```python
from build123d import *

# Parameters (mm, degrees)
SKETCH1_W           = 25.0000008
SKETCH1_H           = 24.00000026
SKETCH1_W_2         = 17.000000544
SKETCH1_H_2         = 16.000000004
BOSS_EXTRUDE1_DEPTH = 2.54
SKETCH2_R           = 1.000000032
CUT_EXTRUDE1_DEPTH  = 2.54


with BuildPart() as part:
    # Sketch1 → Boss-Extrude1 (new body)
    with BuildSketch(Plane.XY):
        Rectangle(SKETCH1_W, SKETCH1_H)
        Rectangle(SKETCH1_W_2, SKETCH1_H_2, mode=Mode.SUBTRACT)
    extrude(amount=BOSS_EXTRUDE1_DEPTH)

    # Sketch2 → Cut-Extrude1 (cut)
    with BuildSketch(Plane.XY.offset(0.635)):
        with Locations((-10.500000336, 9.963437842)):
            Circle(SKETCH2_R)
        with Locations((-10.500000336, -2.536562558)):
            Circle(SKETCH2_R)
        with Locations((10.500000336, 9.963437842)):
            Circle(SKETCH2_R)
        with Locations((10.500000336, -2.536562558)):
            Circle(SKETCH2_R)
    extrude(amount=CUT_EXTRUDE1_DEPTH, mode=Mode.SUBTRACT)


solid = part.part
```
Input: part model. Units: mm. Frame: model coordinates. A direction names the side the tool comes from. Give positions to 0.01 mm unless a question says otherwise; leave off trailing zeros. Order: outer loops, then holes, each group sorted by start corner. A loop starts at its lowest first (then second) coordinate and runs counter-clockwise, first axis right, second up. Notation, with made-up numbers: M -2.75,23 L 5.25,23 A25 cw 5.25,37 Z; hole C 9,49 d7. An arc over 180 degrees is marked long. Return JSON: item names as keys, results as strings.
Item 1: Ray query, probe 1 along Y at (x, z) = (10.5, 2); probe 2 along X at (y, z) = (-0.5, 1.3); probe 3 along Y at (x, z) = (-7.5, 2.05). Return the intervals inside material, ascending.
Solutions:
{"probe 1": "-12 to -3.54, -1.54 to 8.96, 10.96 to 12", "probe 2": "-12.5 to -8.5, 8.5 to 12.5", "probe 3": "-12 to -8, 8 to 12"}
Item 2: Cut plane B-B (x = 1.75). Return loops of the section in (y, z), then the cut area to 3 significant figures.
Solutions:
{"outline": "M -12,0 L -8,0 L -8,2.54 L -12,2.54 Z; M 8,0 L 12,0 L 12,2.54 L 8,2.54 Z", "area": "20.3 mm^2"}
Item 3: Access query for faces 1 (the flat face through (8.5, 0, 1)), 2 (the flat face through (-11, 10, 0.635)), 3 (the flat face through (-9, 0, 2.54)). Directions: +Z, -Z, +X, -X, +Y, -Y. A direction counts if a zero-diameter tool reaches every point of the face in a straight line with its end or side. Return the directions, or none.
Solutions:
{"face 1": "+Z, -Z", "face 2": "+Z", "face 3": "+Z, +X, -X, +Y, -Y"}
Item 4: Pull-direction query (X, two-part tool) for faces 4 (the flat face through (10, 10, 0.635)), 5 (the flat face through (-12.5, 0, 1)), 6 (the flat face through (0, -12, 1)); classes: +X half, -X half, draft (parallel to the pull), parting line (faces both ways), or undercut.
Solutions:
{"face 4": "undercut", "face 5": "-X half", "face 6": "draft"}
Item 5: Cut plane A-A (y = 6). Return loops of the section in (x, z), then the cut area to 3 significant figures.
Solutions:
{"outline": "M -12.5,0 L -8.5,0 L -8.5,2.54 L -12.5,2.54 Z; M 8.5,0 L 12.5,0 L 12.5,2.54 L 8.5,2.54 Z", "area": "20.3 mm^2"}
Item 6: First-contact query: P1, Ø2, axis at x = 1, y = -6.5, coming from the +Z side; P2, Ø1, axis at x = 10.5, y = 10, coming from the +Z side (3 decimals). Flat tips, straight axial feed; report the tip coordinate or a pass-through.
Solutions:
{"P1": "through", "P2": "z = 0.635"}
Item 7: Cut plane D-D (x = 10.5). Return loops of the section in (y, z) (3 decimals), then the cut area to 3 significant figures.
Solutions:
{"outline": "M -12,0 L 12,0 L 12,2.54 L 10.963,2.54 L 10.963,0.635 L 8.963,0.635 L 8.963,2.54 L -1.537,2.54 L -1.537,0.635 L -3.537,0.635 L -3.537,2.54 L -12,2.54 Z", "area": "53.3 mm^2"}
Item 8: Cut plane C-C (z = 2.2). Return loops of the section in (x, y).
Solutions:
{"outline": "M -12.5,-12 L 12.5,-12 L 12.5,12 L -12.5,12 Z; hole C -10.5,-2.54 d2; hole C -10.5,9.96 d2; hole M -8.5,-8 L 8.5,-8 L 8.5,8 L -8.5,8 Z; hole C 10.5,-2.54 d2; hole C 10.5,9.96 d2"}
